```python
from build123d import *
from build123d.topology import SkipClean

# Parameters (mm, degrees)
SKETCH_1_R               = 25
EXTRUDE_1_DEPTH          = 15
SKETCH_2_R               = 22.15
CUT_EXTRUDE_1_DEPTH      = 12.5
SKETCH_3_R               = 18.15
CUT_EXTRUDE_2_DEPTH      = 12.5
EXTRUDE_2_DEPTH          = 15
FILLET_1_R               = 8
CUT_EXTRUDE_START        = -15
SKETCH_5_R               = 1.5
CUT_EXTRUDE_3_DEPTH      = 15
SKETCH_6_R               = 3
CUT_EXTRUDE_4_DEPTH      = 2
PATTERN_CIRCULAR_1_COUNT = 4
FILLET_2_R               = 2


with BuildPart() as part:
    # 草图1 → 凸台-拉伸1 (new body)
    with BuildSketch(Plane(origin=(0, 0, 0), x_dir=(1, 0, 0), z_dir=(0, 1, 0))):
        with Locations(Location((0, 0, 0), (0, 0, 270))):
            Circle(SKETCH_1_R)
    extrude(amount=EXTRUDE_1_DEPTH)

    # 草图2 → 切除-拉伸1 (cut)
    with BuildSketch(Plane(origin=(0, 15, 0), x_dir=(1, 0, 0), z_dir=(0, 1, 0))):
        with Locations(Location((0, 0, 0), (0, 0, 270))):
            Circle(SKETCH_2_R)
    extrude(amount=-CUT_EXTRUDE_1_DEPTH, mode=Mode.SUBTRACT)

    # 草图3 → 切除-拉伸2 (cut)
    with BuildSketch(Plane(origin=(0, 2.5, 0), x_dir=(1, 0, 0), z_dir=(0, 1, 0))):
        with Locations(Location((0, 0, 0), (0, 0, 270))):
            Circle(SKETCH_3_R)
    extrude(amount=-CUT_EXTRUDE_2_DEPTH, mode=Mode.SUBTRACT)

    # 草图4 → 凸台-拉伸2 (add)
    with BuildSketch(Plane(origin=(0, 0, 0), x_dir=(1, 0, 0), z_dir=(0, 1, 0))):
        with BuildLine():
            Line((0, 25), (-25, 25))
            Line((-25, 25), (-25, 2.6e-08))
            ThreePointArc((-25, 2.6e-08), (-23.301207713, 9.058350794), (-18.435702489, 16.885641052))
            ThreePointArc((-18.435702489, 16.885641052), (-19.445436483, 19.445436483), (-16.885641052, 18.435702489))
            ThreePointArc((-16.885641052, 18.435702489), (-9.058350782, 23.301207718), (0, 25))
        make_face()
        with BuildLine():
            Line((25, 25), (0, 25))
            ThreePointArc((0, 25), (9.210354363, 23.241544108), (17.125028574, 18.213549801))
            ThreePointArc((17.125028574, 18.213549801), (19.682469279, 19.438809921), (18.425448396, 16.896829626))
            ThreePointArc((18.425448396, 16.896829626), (23.298457137, 9.065423048), (25, 0))
            Line((25, 0), (25, 25))
        make_face()
        with BuildLine():
            ThreePointArc((-18.213549801, -17.125028574), (-23.241544113, -9.210354351), (-25, 2.6e-08))
            Line((-25, 2.6e-08), (-25, -25))
            Line((-25, -25), (-5.8e-08, -25))
            ThreePointArc((-5.8e-08, -25), (-9.065423076, -23.298457126), (-16.896829626, -18.425448396))
            ThreePointArc((-16.896829626, -18.425448396), (-19.438809921, -19.682469279), (-18.213549801, -17.125028574))
        make_face()
        with BuildLine():
            Line((25, -25), (25, 0))
            ThreePointArc((25, 0), (23.22561674, -9.250444694), (18.154341838, -17.18778265))
            ThreePointArc((18.154341838, -17.18778265), (19.675883861, -19.675883861), (17.18778265, -18.154341838))
            ThreePointArc((17.18778265, -18.154341838), (9.250444666, -23.225616751), (-5.8e-08, -25))
            Line((-5.8e-08, -25), (25, -25))
        make_face()
    extrude(amount=EXTRUDE_2_DEPTH)

    # 圆角1
    fillet_1_edges = [part.edges().sort_by_distance(p)[0] for p in [
        (-25, 7.5, -25),
        (25, 7.5, -25),
        (-25, 7.5, 25),
        (25, 7.5, 25),
    ]]
    fillet(fillet_1_edges, radius=FILLET_1_R)

    # 草图5 → 切除-拉伸3 (cut)
    with BuildSketch(Plane(origin=(0, 15, 0), x_dir=(1, 0, 0), z_dir=(0, 1, 0)).offset(CUT_EXTRUDE_START)):
        with Locations(Location((-18.384776311, 18.384776311, 0), (0, 0, 270))):
            Circle(SKETCH_5_R)
        with Locations(Location((18.615223689, 18.384776311, 0), (0, 0, 270))):
            Circle(SKETCH_5_R)
        with Locations(Location((18.615223689, -18.615223689, 0), (0, 0, 270))):
            Circle(SKETCH_5_R)
        with Locations(Location((-18.384776311, -18.615223689, 0), (0, 0, 270))):
            Circle(SKETCH_5_R)
    extrude(amount=CUT_EXTRUDE_3_DEPTH, mode=Mode.SUBTRACT)

    # 草图6 → 切除-拉伸4 (cut)
    with BuildSketch(Plane(origin=(0, 15, 0), x_dir=(1, 0, 0), z_dir=(0, 1, 0))):
        with Locations(Location((-18.384776311, 18.384776311, 0), (0, 0, 270))):
            Circle(SKETCH_6_R)
    cut_extrude_4 = extrude(amount=-CUT_EXTRUDE_4_DEPTH, mode=Mode.SUBTRACT)

    # 阵列(圆周)1: 切除-拉伸4 ×4 about axis
    with SkipClean():  # the faces are left unmerged after this step: merging them gives an invalid solid
        pattern_circular_1_axis = Axis((0, 0, 0), (0, 1, 0))
        for i in range(1, PATTERN_CIRCULAR_1_COUNT):
            add(cut_extrude_4.rotate(pattern_circular_1_axis, i * 360 / PATTERN_CIRCULAR_1_COUNT), mode=Mode.SUBTRACT)

    # 圆角2
    # the kernel refuses this fillet: 2 mm, written as the material it takes off along each edge
    with BuildSketch(Plane(origin=(0, 15, 0), x_dir=(0, 0, 1), z_dir=(-1, 0, 0))) as fillet_2_piece_1:
        with BuildLine():
            CenterArc((22.15 + FILLET_2_R, -FILLET_2_R), FILLET_2_R, 90, 90)
            Line((22.15, -FILLET_2_R), (22.15, 0))
            Line((22.15, 0), (22.15 + FILLET_2_R, 0))
        make_face()
    revolve(axis=Axis((0, 15, 0), (0, 1, 0)), mode=Mode.SUBTRACT)


solid = part.part
```
CAD build for the part. Positions are in the model's coordinates, mm. A direction names the side the tool comes from. Round coordinates to 2 decimals unless told otherwise and drop trailing zeros. Loops run counter-clockwise (first coordinate to the right, second up) from the corner with the lowest first, then second, coordinate; pieces in that order, holes last. Notation, with made-up numbers: M -38,-35.75 L -29,-35.75 A22 ccw -29,0.25 Z; hole C 0,-8 d11. An arc over 180 degrees is marked long. Return JSON: item names as keys, results as strings. Group by question number.
(1) Tool access for faces 1 (the cylindrical face through (-20.21, 14.014, -20.765)), 2 (the cylindrical face through (-11.044, 1.268, -14.403)): list every direction of +Z, -Z, +X, -X, +Y, -Y with a clear straight run to the whole face (end or side of a thin tool).
(2) Mould opens along X. For faces 3 (the flat face through (18, 13, 17)), 4 (the cylindrical face through (22.594, 7.605, -22.719)), 5 (the flat face through (0, 7, -25)), 6 (the flat face through (-25, 7, 0)) say: +X half, -X half, draft (parallel to the pull), parting line (faces both ways), or undercut.
(3) Saw through at A-A, the plane x = 0. List the corners of the cut face in (y, z), and give its area (3 significant figures).
(4) Saw through at B-B, the plane z = 0. List the corners of the cut face in (x, y).
(5) Drop a flat-ended pin along its axis: P1, Ø3.5, axis at x = -18.38, z = -18.38, coming from the +Y side. Give the stop position or say it passes through.
(6) Saw through at C-C, the plane y = 7.25. List the corners of the cut face in (x, z), and give its area (3 significant figures).
(7) Wall check: probe 1 along X at (y, z) = (8.5, 17.5); probe 2 along Z at (x, y) = (18, 10.75); probe 3 along Y at (x, z) = (21, 5). Give the ranges that are in metal, low to high. Write a range as [from, to].
Answer list:
{
 "1": {"face 1": "+Y", "face 2": "+Y, -Y"},
 "2": {"face 3": "undercut", "face 4": "+X half", "face 5": "draft", "face 6": "-X half"},
 "3": {"outline": "M 0,-25 L 15,-25 L 15,-24.15 A2 ccw 13,-22.15 L 2.5,-22.15 L 2.5,-18.15 L 0,-18.15 Z; M 0,18.15 L 2.5,18.15 L 2.5,22.15 L 13,22.15 A2 ccw 15,24.15 L 15,25 L 0,25 Z", "area": "104 mm2"},
 "4": {"outline": "M -25,0 L -18.15,0 L -18.15,2.5 L -22.15,2.5 L -22.15,13 A2 ccw -24.15,15 L -25,15 Z; M 18.15,0 L 25,0 L 25,15 L 24.15,15 A2 ccw 22.15,13 L 22.15,2.5 L 18.15,2.5 Z"},
 "5": {"P1": "y = 13"},
 "6": {"outline": "M -25,-17 A8 ccw -17,-25 L 17,-25 A8 ccw 25,-17 L 25,17 A8 ccw 17,25 L -17,25 A8 ccw -25,17 Z; hole C 0,0 d44.3; hole C -18.38,-18.38 d3; hole C -18.38,18.62 d3; hole C 18.62,-18.38 d3; hole C 18.62,18.62 d3", "area": "875 mm2"},
 "7": {"probe 1": "[-24.98, -19.39], [-17.38, -13.58], [13.58, 17.61], [19.62, 24.98]", "probe 2": "[-24.94, -19.75], [-17.02, -12.91], [12.91, 17.25], [19.98, 24.94]", "probe 3": "[0, 2.5]"}
}
